```python
from build123d import *

# Parameters (mm, degrees)
F0_W     = 90.5727781355
F0_H     = 92.5153568387
F1_DEPTH = 69.85
F2_T     = -2.54
F3_W     = 90.5727781355
F3_H     = 69.85
F4_DEPTH = 13.716
F5_W     = 7.770318538
F5_H     = 7.2846729308
F5_H_2   = 7.5274929404
F6_DEPTH = 90.5737781355


with BuildPart() as f1:
    # F0 (on Front) → F1 (new body)
    with BuildSketch(Plane.XZ):
        with Locations((1.9425805658, -7.1646422148)):
            Rectangle(F0_W, F0_H)
    extrude(amount=-F1_DEPTH)

    # F2
    f2_openings = [f1.faces().sort_by_distance(p)[0] for p in [
        (1.942581, 0, -7.164642),
    ]]
    offset(amount=F2_T, openings=f2_openings)

    # F3 (on face) → F4 (cut)
    with BuildSketch(Plane.XY.offset(39.0930362046)):
        with Locations((1.9425805658, 34.925)):
            Rectangle(F3_W, F3_H)
    extrude(amount=-F4_DEPTH, mode=Mode.SUBTRACT)

    # F5 (on face) → F6 (cut, through all)
    with BuildSketch(Plane(origin=(-43.343808502, 0, 0), x_dir=(0, -1, 0), z_dir=(-1, 0, 0))):
        with Locations((-10.5627775192, 16.9961908832)):
            Rectangle(F5_W, F5_H)
        with Locations((-61.5554954857, -45.5305911601)):
            Rectangle(F5_W, F5_H_2)
    extrude(amount=-F6_DEPTH, mode=Mode.SUBTRACT)


solid = f1.part
```
The listing builds one solid part. Answer for the finished solid, in the listing's coordinates (mm). A direction names the side the tool comes from. Coordinates: 2 decimals unless noted, no trailing zeros. Write each loop counter-clockwise with the first axis right and the second up, starting at its lowest first coordinate (ties: lowest second). Pieces come first, ordered by that corner, then holes. Notation, with made-up numbers: (-30, 82.25) - (1, 82.25) arc R22 cw to (1, 108.25) - close; hole circle Ø8 at (45.5, -17). An arc over 180 degrees is marked (long way). Return JSON: item names as keys, results as strings. Group by question number.
Q1. Which of the six approach directions +Z, -Z, +X, -X, +Y, -Y give full straight-line access (tool end or side, diameter ignored) to faces 4 (the flat face through (-42, 62, -41.767)), 5 (the flat face through (1, 69.85, -13)), 6 (the flat face through (-40.804, 33, -13))?
Q2. For a pull along X with two mould halves and no side action, classify faces 1 (the flat face through (47.229, 34, -15)), 2 (the flat face through (-42, 57.67, -46)), 3 (the flat face through (1, 33, -50.882)) as +X half, -X half, draft (parallel to the pull), parting line (faces both ways), or undercut.
Q3. Flat-ended cylindrical pins translate along their axes: pin 1 Ø4 at (x, y) = (34.5, 11.5) entering from +Z; pin 2 Ø12 at (x, z) = (32.5, 0) entering from -Y. Find the tip coordinate at first contact, or state that the pin passes through.
Q4. The part is cut by section A-A on y = 63. Write down the section's boundary in (x, z).
Q5. The part is cut by section C-C on y = 17.5. Write down the section's boundary in (x, z).
Q6. Find the intervals of material crossed by line 1 along X through (y, z) = (59.5, -39); line 2 along Y through (x, z) = (-0.5, 2.5); line 3 along Z through (x, y) = (-17.5, 58), in increasing order. Write a range as [from, to].
Q7. The part is cut by section B-B on z = 7. Write down the section's boundary in (x, y), and give its area (3 significant figures).
Q8. The part is cut by section D-D on x = 20. Write down the section's boundary in (y, z).
Evaluation:
{
 "1": {"face 4": "+X, -X", "face 5": "+Z, -Z, +X, -X, +Y", "face 6": "+Z, -Y"},
 "2": {"face 1": "+X half", "face 2": "draft", "face 3": "undercut"},
 "3": {"pin 1": "stops at z = -50.88", "pin 2": "stops at y = 67.31"},
 "4": {"outline": "(-43.34, -53.42) - (47.23, -53.42) - (47.23, -49.29) - (44.69, -49.29) - (44.69, -50.88) - (-40.8, -50.88) - (-40.8, -49.29) - (-43.34, -49.29) - close; (-43.34, -41.77) - (-40.8, -41.77) - (-40.8, 25.38) - (-43.34, 25.38) - close; (44.69, -41.77) - (47.23, -41.77) - (47.23, 25.38) - (44.69, 25.38) - close"},
 "5": {"outline": "(-43.34, -53.42) - (47.23, -53.42) - (47.23, 25.38) - (44.69, 25.38) - (44.69, -50.88) - (-40.8, -50.88) - (-40.8, 25.38) - (-43.34, 25.38) - close"},
 "6": {"line 1": "x = [-43.34, -40.8], [44.69, 47.23]", "line 2": "y = [67.31, 69.85]", "line 3": "z = [-53.42, -50.88]"},
 "7": {"outline": "(-43.34, 0) - (-40.8, 0) - (-40.8, 67.31) - (44.69, 67.31) - (44.69, 0) - (47.23, 0) - (47.23, 69.85) - (-43.34, 69.85) - close", "area": "572 mm2"},
 "8": {"outline": "(0, -53.42) - (69.85, -53.42) - (69.85, 25.38) - (67.31, 25.38) - (67.31, -50.88) - (0, -50.88) - close"}
}
